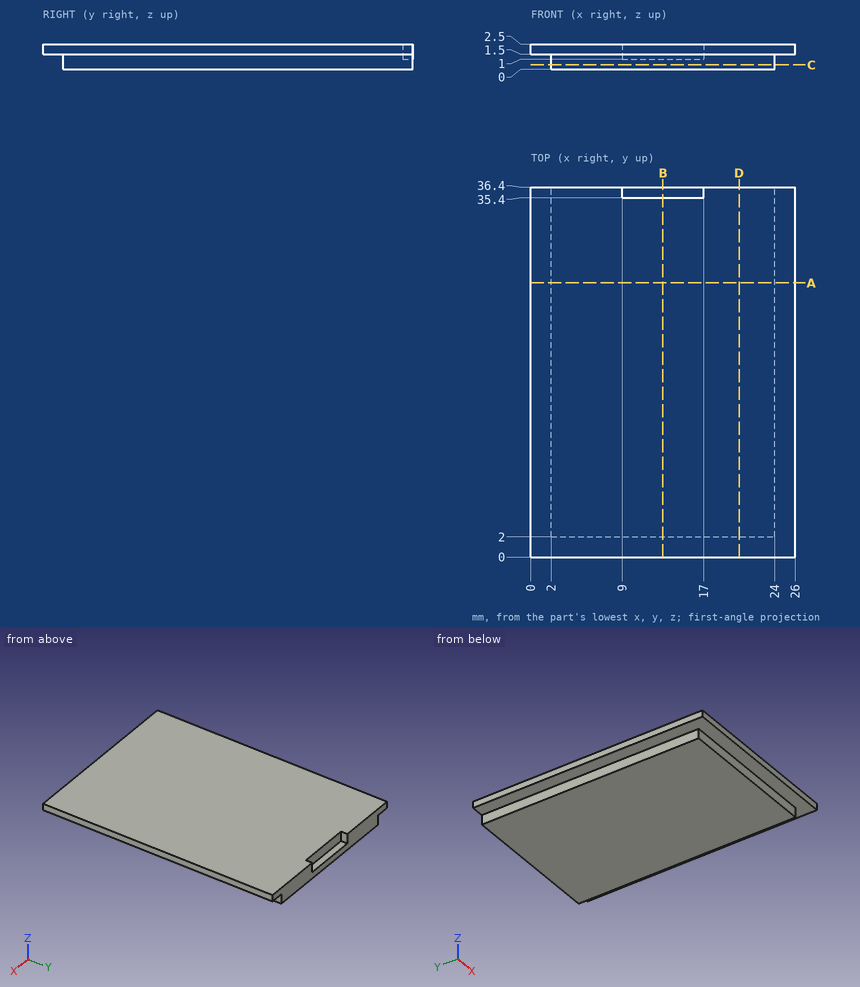
The figure shows three views and two pictorial views of one solid part (mm, origin at its lowest corner). Answer the questions. Round coordinates to 2 decimals unless told otherwise and drop trailing zeros. Loops run counter-clockwise (first coordinate to the right, second up) from the corner with the lowest first, then second, coordinate; pieces in that order, holes last. Notation, with made-up numbers: M -37,17 L 1,17 A13 cw 1,28 Z; hole C -32,50 d9. An arc over 180 degrees is marked long. Use CSV: the item, a comma, the result in double quotes.
Q1. This flat-tipped pin is pushed along its axis until it touches: pin 1 (1.1 mm diameter, centred on y = 36, z = 1.5, fed in from -X). Where does it stop, or does it pass through?
Determined:
pin 1,"x = 0"
Q2. Section B-B, the plane x = 13 is taken. Determine the outline of the cut face in (y, z).
Determined:
outline,"M 0,1.5 L 2,1.5 L 2,0 L 36.4,0 L 36.4,1 L 35.4,1 L 35.4,2.5 L 0,2.5 Z"
Q3. Section C-C, the plane z = 0.45 is taken. Determine the outline of the cut face in (x, y), then the cut area to 3 significant figures.
Determined:
outline,"M 2,2 L 24,2 L 24,36.4 L 2,36.4 Z"
area,"757 mm2"
Q4. Section A-A, the plane y = 27 is taken. Determine the outline of the cut face in (x, z), then the cut area to 3 significant figures.
Determined:
outline,"M 0,1.5 L 2,1.5 L 2,0 L 24,0 L 24,1.5 L 26,1.5 L 26,2.5 L 0,2.5 Z"
area,"59.0 mm2"
Q5. Consider L1, parallel to X at y = 17, z = 0.75; L2, parallel to Y at x = 14.75, z = 1.4; L3, parallel to Z at x = 1.5, y = 20. Determine where each line is inside the solid, lowest interval first.
Determined:
L1,"2 to 24"
L2,"2 to 35.4"
L3,"1.5 to 2.5"
Q6. Section D-D, the plane x = 20.5 is taken. Determine the outline of the cut face in (y, z), then the cut area to 3 significant figures.
Determined:
outline,"M 0,1.5 L 2,1.5 L 2,0 L 36.4,0 L 36.4,2.5 L 0,2.5 Z"
area,"88.0 mm2"
